from build123d import *

# Parameters (mm, degrees)
CROQUIS2_R              = 5
SALIENTE_EXTRUIR1_DEPTH = 250
SALIENTE_EXTRUIR2_DEPTH = 2.5
CROQUIS11_R             = 4.5
SALIENTE_EXTRUIR3_DEPTH = 19
CORTAR_EXTRUIR1_REACH   = 276.178
CROQUIS12_R             = 3


with BuildPart() as part:
    # Croquis2 → Saliente-Extruir1 (new body)
    with BuildSketch(Plane(origin=(0, 0, 0), x_dir=(1, 0, 0), z_dir=(0, 1, 0))):
        with Locations(Location((-11.975261547, 2.214603163, 0), (0, 0, 270))):
            Circle(CROQUIS2_R)
    extrude(amount=SALIENTE_EXTRUIR1_DEPTH)

    # Cortar-Recubrir1: read off the stored shape, not the designer's step
    # Cortar-Recubrir1: loft between two sections, ruled curve by curve
    cortar_recubrir1_from = [
        Edge.make_bspline([(-12.756084652, 7, -1.589850989), (-14.005589, 7, -3.151497198), (-12.443942791, 7, -4.401001547), (-11.194438443, 7, -2.839355337), (-9.944934094, 7, -1.277709127), (-11.506580304, 7, -0.028204779), (-12.756084652, 7, -1.589850989)], [0, 0, 0, 0, 0.5, 0.5, 0.5, 1, 1, 1, 1], 3, [1, 0.333333333, 0.333333333, 1, 0.333333333, 0.333333333, 1]),
    ]
    cortar_recubrir1_to = [
        Edge.make_bspline([(-14.386979714, 0, 0.976574595), (-20.76933523, 0, -3.846861738), (-15.945898897, 0, -10.229217255), (-9.563543381, 0, -5.405780921), (-3.181187864, 0, -0.582344588), (-8.004624198, 0, 5.800010929), (-14.386979714, 0, 0.976574595)], [0, 0, 0, 0, 0.5, 0.5, 0.5, 1, 1, 1, 1], 3, [1, 0.333333333, 0.333333333, 1, 0.333333333, 0.333333333, 1]),
    ]
    cortar_recubrir1 = Solid(Shell([*[Face.make_surface_from_curves(cortar_recubrir1_from[k], cortar_recubrir1_to[k]) for k in range(1)], Face(Wire(cortar_recubrir1_from)), Face(Wire(cortar_recubrir1_to))]))
    add(cortar_recubrir1, mode=Mode.SUBTRACT)

    # Croquis7 → Saliente-Extruir2 (add)
    with BuildSketch(Plane(origin=(0, 250, 0), x_dir=(1, 0, 0), z_dir=(0, 1, 0))):
        with BuildLine():
            Line((-30.826612899, 8.705100234), (-12.380666953, 9.703638245))
            ThreePointArc((-12.380666953, 9.703638245), (-4.475261547, 2.214603163), (-12.380666953, -5.274431919))
            Line((-12.380666953, -5.274431919), (-30.826612899, -4.275893908))
            ThreePointArc((-30.826612899, -4.275893908), (-36.975261547, 2.214603163), (-30.826612899, 8.705100234))
        make_face()
    extrude(amount=SALIENTE_EXTRUIR2_DEPTH)

    # Cortar-Recubrir2: read off the stored shape, not the designer's step
    # Cortar-Recubrir2: loft between two sections, ruled curve by curve
    cortar_recubrir2_from = [
        Edge.make_bspline([(-12.878746512, 244.5, -2.643222947), (-13.735986079, 244.5, -0.836253018), (-11.92901615, 244.5, 0.02098655), (-11.071776583, 244.5, -1.785983379), (-10.214537015, 244.5, -3.592953308), (-12.021506944, 244.5, -4.450192876), (-12.878746512, 244.5, -2.643222947)], [0, 0, 0, 0, 0.5, 0.5, 0.5, 1, 1, 1, 1], 3, [1, 0.333333333, 0.333333333, 1, 0.333333333, 0.333333333, 1]),
    ]
    cortar_recubrir2_to = [
        Edge.make_bspline([(-14.629528251, 252.5, 0.066814876), (-10.066692174, 252.5, 5.375348283), (-4.758158767, 252.5, 0.812512206), (-9.320994844, 252.5, -4.496021201), (-13.883830921, 252.5, -9.804554608), (-19.192364328, 252.5, -5.241718531), (-14.629528251, 252.5, 0.066814876)], [0, 0, 0, 0, 0.5, 0.5, 0.5, 1, 1, 1, 1], 3, [1, 0.333333333, 0.333333333, 1, 0.333333333, 0.333333333, 1]),
    ]
    cortar_recubrir2 = Solid(Shell([*[Face.make_surface_from_curves(cortar_recubrir2_from[k], cortar_recubrir2_to[k]) for k in range(1)], Face(Wire(cortar_recubrir2_from)), Face(Wire(cortar_recubrir2_to))]))
    add(cortar_recubrir2, mode=Mode.SUBTRACT)

    # Croquis11 → Saliente-Extruir3 (add)
    with BuildSketch(Plane(origin=(0, 252.5, 0), x_dir=(1, 0, 0), z_dir=(0, 1, 0))):
        with Locations(Location((-30.475261547, 2.214603163, 0), (0, 0, 270))):
            Circle(CROQUIS11_R)
    extrude(amount=SALIENTE_EXTRUIR3_DEPTH)

    # Croquis12 → Cortar-Extruir1 (cut, up to next)
    with BuildSketch(Plane(origin=(0, 271.5, 0), x_dir=(1, 0, 0), z_dir=(0, 1, 0)), mode=Mode.PRIVATE) as cortar_extruir1_sk1:
        with Locations(Location((-30.475261547, 2.214603163, 0), (0, 0, 270))):
            Circle(CROQUIS12_R)
    cortar_extruir1_tool1 = extrude(cortar_extruir1_sk1.sketch, amount=-CORTAR_EXTRUIR1_REACH, mode=Mode.PRIVATE) & part.part
    add(cortar_extruir1_tool1.solids().sort_by_distance((-30.475262, 271.5, -2.214603))[0], mode=Mode.SUBTRACT)


solid = part.part
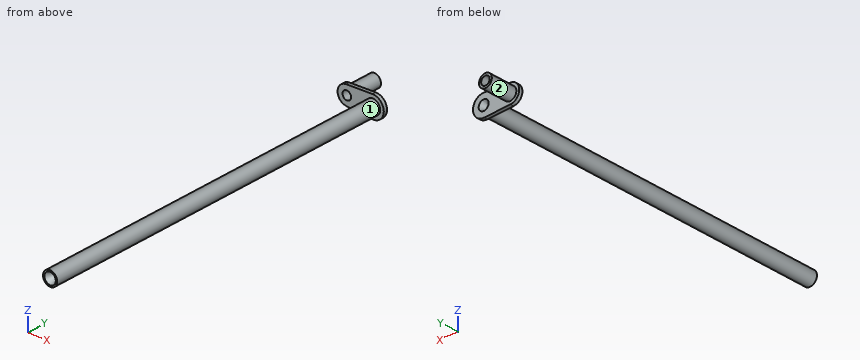
Model file for the job. Use its own axes, mm. Face numbers are marked on the shaded views. A direction names the side the tool comes from. Give positions to 0.01 mm unless a question says otherwise; leave off trailing zeros. Order: outer loops, then holes, each group sorted by start corner. A loop starts at its lowest first (then second) coordinate and runs counter-clockwise, first axis right, second up. Notation, with made-up numbers: (50, 55.5) - (82, 55.5) arc R29 cw to (82, 78.5) - close; hole circle Ø5 at (36.5, 53). An arc over 180 degrees is marked (long way). One line per item, written item: value.
Item 1: Tool access for the marked faces 1 and 2: list every direction of +Z, -Z, +X, -X, +Y, -Y with a clear straight run to the whole face (end or side of a thin tool).
Response values:
face 1: -Y
face 2: +Y
Item 2: Wall check: line 1 (Y direction, x = -29, z = -6.25); line 2 (X direction, y = 139.5, z = -2.75); line 3 (Y direction, x = -32.5, z = -7). Give the ranges that are in metal, low to high.
Response values:
line 1: 250 to 271.5
line 2: -16.95 to -7
line 3: 250 to 252.5
Item 3: Slice it at A-A (x = -19.5). List the corners of the cut face in (y, z), then the cut area to 3 significant figures.
Response values:
outline: (250, -9.32) - (252.5, -9.32) - (252.5, 4.89) - (250, 4.89) - close
area: 35.5 mm2
Item 4: Slice it at B-B (y = 37). List the corners of the cut face in (x, z), then the cut area to 3 significant figures.
Response values:
outline: circle Ø10 at (-11.98, -2.21)
area: 78.5 mm2
Item 5: Pin check, flat tips, straight feed: pin 1 Ø1.6 at (x, z) = (-12, -2.5) entering from -Y; pin 2 Ø4.5 at (x, z) = (-24, -2.5) entering from -Y; pin 3 Ø7.5 at (x, z) = (-26, 0) entering from +Y; pin 4 Ø8 at (y, z) = (193.5, -7.5) entering from -X. Stop position of each tip, or through.
Response values:
pin 1: y = 6.79
pin 2: y = 250
pin 3: y = 271.5
pin 4: x = -16.81
